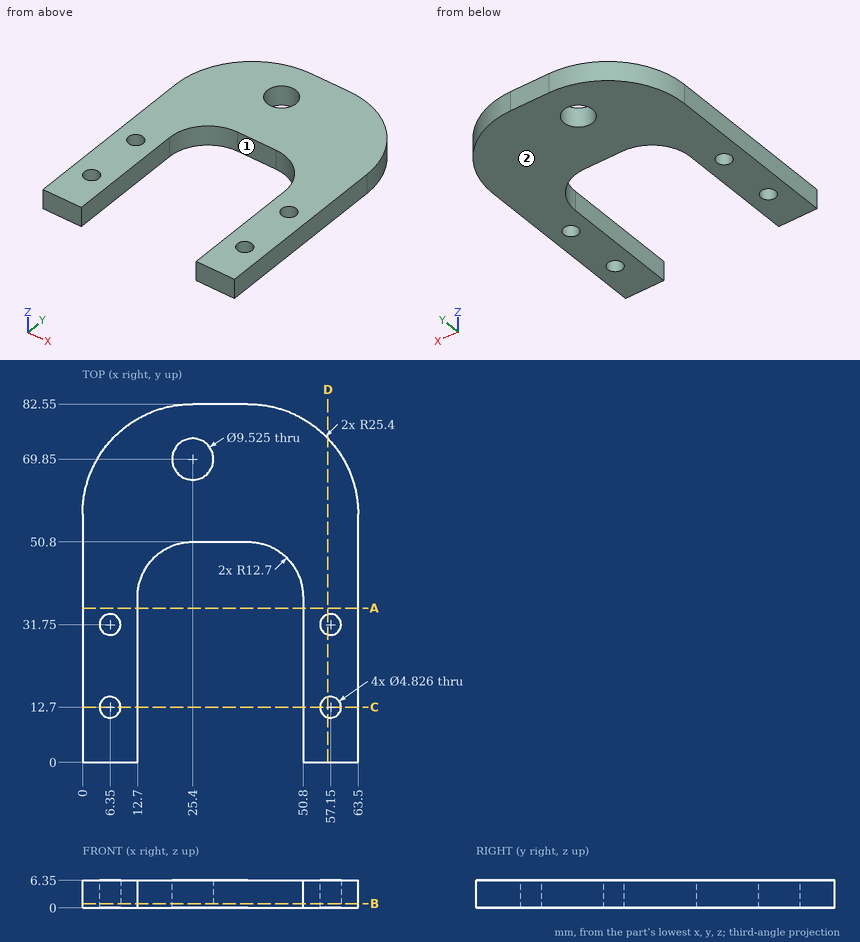
Answer from the drawing. Dimensions are ordinates in mm from the lowest x, y and z of the part. A direction names the side the tool comes from. Round coordinates to 2 decimals unless told otherwise and drop trailing zeros. Write each loop counter-clockwise with the first axis right and the second up, starting at its lowest first coordinate (ties: lowest second). Pieces come first, ordered by that corner, then holes. Notation, with made-up numbers: (-20.5, 17.5) -> (18.5, 17.5) arc R24 cw to (18.5, 56.5) -> close; hole circle Ø9 at (82, 14). An arc over 180 degrees is marked (long way). Answer in a Markdown table with one row per item. Add a question column.
1) Find section C-C, the plane y = 12.7. Determine the outline of the cut face in (x, z), and give its area (4 significant figures).
2) Find section B-B, the plane z = 1. State how many separate pieces and enclosed holes the cut face has, and give its area (3 significant figures).
3) Which of the six approach directions +Z, -Z, +X, -X, +Y, -Y give full straight-line access (tool end or side, diameter ignored) to the marked faces 1 and 2?
4) Consider line 1 (X direction, y = 24, z = 3); line 2 (Y direction, x = 56, z = 1.5); line 3 (Y direction, x = 6.35, z = 2.75). Determine where each line is inside the solid, lowest interval first.
5) Find section D-D, the plane x = 56.5. Determine the outline of the cut face in (y, z).
6) Find section A-A, the plane y = 35.5. Determine the outline of the cut face in (x, z), and give its area (3 significant figures).
Findings below:
| question | item | result |
|---|---|---|
| 1 | outline | (0, 0) -> (3.94, 0) -> (3.94, 6.35) -> (0, 6.35) -> close; (8.76, 0) -> (12.7, 0) -> (12.7, 6.35) -> (8.76, 6.35) -> close; (50.8, 0) -> (54.74, 0) -> (54.74, 6.35) -> (50.8, 6.35) -> close; (59.56, 0) -> (63.5, 0) -> (63.5, 6.35) -> (59.56, 6.35) -> close |
| 1 | area | 100.0 mm² |
| 2 | separate pieces | 1 |
| 2 | enclosed holes | 5 |
| 2 | area | 2,950 mm² |
| 3 | face 1 | +Z, -Z, -Y |
| 3 | face 2 | -Z, +X, -X, +Y, -Y |
| 4 | line 1 | 0 to 12.7, 50.8 to 63.5 |
| 4 | line 2 | 0 to 10.58, 14.82 to 29.63, 33.87 to 75.17 |
| 4 | line 3 | 0 to 10.29, 15.11 to 29.34, 34.16 to 73.95 |
| 5 | outline | (0, 0) -> (10.38, 0) -> (10.38, 6.35) -> (0, 6.35) -> close; (15.02, 0) -> (29.43, 0) -> (29.43, 6.35) -> (15.02, 6.35) -> close; (34.07, 0) -> (74.66, 0) -> (74.66, 6.35) -> (34.07, 6.35) -> close |
| 6 | outline | (0, 0) -> (12.7, 0) -> (12.7, 6.35) -> (0, 6.35) -> close; (50.8, 0) -> (63.5, 0) -> (63.5, 6.35) -> (50.8, 6.35) -> close |
| 6 | area | 161 mm² |
